Here's how the part is built. I have some questions about the finished solid (model axes, mm). Face numbers are marked on the shaded views. Round coordinates to 2 decimals unless told otherwise and drop trailing zeros. Loops run counter-clockwise (first coordinate to the right, second up) from the corner with the lowest first, then second, coordinate; pieces in that order, holes last. Notation, with made-up numbers: M 38.5,61 L 90.5,61 A26 cw 90.5,91 Z; hole C -21.5,63 d4. An arc over 180 degrees is marked long. Use a Markdown table: item, result.
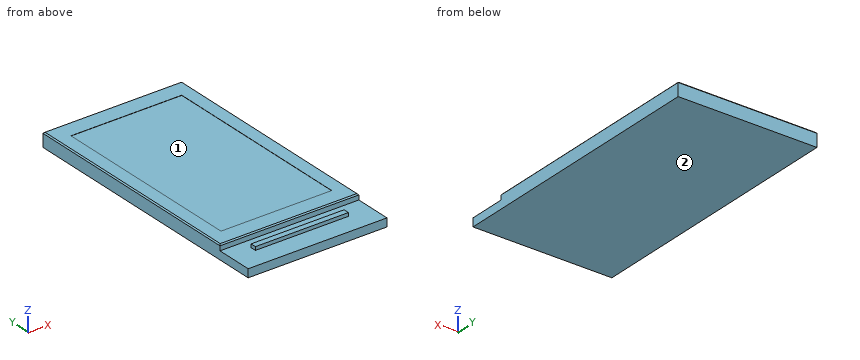
```python
from build123d import *

# Parameters (mm, degrees)
SKETCH_W     = 12.13
SKETCH_H     = 23.6
PAD_DEPTH    = 0.72
SKETCH001_W  = 12.13
SKETCH001_H  = 20.36
PAD001_DEPTH = 0.5
SKETCH002_W  = 8.13
SKETCH002_H  = 0.5
PAD002_DEPTH = 0.3
SKETCH003_W  = 9.68
SKETCH003_H  = 17.26
POCKET_DEPTH = 0.02
CHAMFER_SIZE = 0.1


with BuildPart() as part:
    # Sketch → Pad (new body)
    with BuildSketch(Plane.XY):
        with Locations((6.065, 11.8)):
            Rectangle(SKETCH_W, SKETCH_H)
    extrude(amount=PAD_DEPTH)

    # Sketch001 (on Face6 of Pad) → Pad001 (join)
    with BuildSketch(Plane.XY.offset(0.72)):
        with Locations((6.065, 13.42)):
            Rectangle(SKETCH001_W, SKETCH001_H)
    extrude(amount=PAD001_DEPTH)

    # Sketch002 (on Face5 of Pad001) → Pad002 (join)
    with BuildSketch(Plane.XY.offset(0.72)):
        with Locations((6.065, 2.05)):
            Rectangle(SKETCH002_W, SKETCH002_H)
    extrude(amount=PAD002_DEPTH)

    # Sketch003 (on Face15 of Pad002) → Pocket (cut)
    with BuildSketch(Plane.XY.offset(1.22)):
        with Locations((6.065, 13.37)):
            Rectangle(SKETCH003_W, SKETCH003_H)
    extrude(amount=-POCKET_DEPTH, mode=Mode.SUBTRACT)

    # Chamfer
    chamfer_edges = [part.edges().sort_by_distance(p)[0] for p in [
        (6.065, 23.6, 1.22),
        (0, 13.42, 1.22),
        (6.065, 3.24, 1.22),
        (12.13, 13.42, 1.22),
    ]]
    chamfer(chamfer_edges, length=CHAMFER_SIZE)


solid = part.part
```
Q1. I need wall thicknesses on line 1 (Y direction, x = 6.75, z = 0.8); line 2 (Z direction, x = 1.75, y = 6); line 3 (Y direction, x = 9, z = 1.1). Which ranges of each line are inside material? Lowest first, please. Write a range as from..to.
Return value:
| item | result |
|---|---|
| line 1 | y = 1.8..2.3, 3.24..23.6 |
| line 2 | z = 0..1.2 |
| line 3 | y = 3.24..23.6 |
Q2. We'd pull the mould along Y, two halves only. Please class the marked faces 1 and 2: pulls with the +Y half, pulls with the -Y half, needs draft (parallel to the pull), parting line crosses it, or undercut.
Return value:
| item | result |
|---|---|
| face 1 | undercut |
| face 2 | needs draft |
Q3. Imagine slicing it at B-B, the plane y = 2.75. Please give me the cut outline in (x, z).
Return value:
| item | result |
|---|---|
| outline | M 0,0 L 12.13,0 L 12.13,0.72 L 0,0.72 Z |
Q4. Will these pins go through, and if not, where does the flat tip stop? P1, Ø0.6, axis at x = 6.5, y = 2, coming from the +Z side; P2, Ø1.5, axis at x = 2.5, y = 18, coming from the +Z side.
Return value:
| item | result |
|---|---|
| P1 | stops at z = 1.02 |
| P2 | stops at z = 1.2 |
